from build123d import *

# Parameters (mm, degrees)
ESBO_O1_R                = 12.1
ESBO_O1_R_2              = 1.6
RESSALTO_EXTRUS_O1_DEPTH = 6
FILETE2_R                = 5
FILETE3_R                = 4


with BuildPart() as part:
    # Esboço1 → Ressalto-extrusão1 (new body)
    with BuildSketch(Plane.XY):
        with BuildLine():
            Line((-25, 4), (-16.625582697, 4))
            ThreePointArc((-16.625582697, 4), (0, 17.1), (16.625582697, 4))
            Line((16.625582697, 4), (25, 4))
            Line((25, 4), (25, -4))
            Line((25, -4), (16.625582697, -4))
            ThreePointArc((16.625582697, -4), (0, -17.1), (-16.625582697, -4))
            Line((-16.625582697, -4), (-25, -4))
            Line((-25, -4), (-25, 4))
        make_face()
        Circle(ESBO_O1_R, mode=Mode.SUBTRACT)
        with Locations((-21, 0)):
            Circle(ESBO_O1_R_2, mode=Mode.SUBTRACT)
        with Locations((21, 0)):
            Circle(ESBO_O1_R_2, mode=Mode.SUBTRACT)
    extrude(amount=RESSALTO_EXTRUS_O1_DEPTH)

    # Filete2
    filete2_edges = [part.edges().sort_by_distance(p)[0] for p in [
        (-16.625582697, 4, 3),
        (16.625582697, 4, 3),
        (16.625582697, -4, 3),
        (-16.625582697, -4, 3),
    ]]
    fillet(filete2_edges, radius=FILETE2_R)

    # Filete3
    filete3_edges = [part.edges().sort_by_distance(p)[0] for p in [
        (25, -4, 3),
        (25, 4, 3),
        (-25, -4, 3),
        (-25, 4, 3),
    ]]
    fillet(filete3_edges, radius=FILETE3_R - 0.0001)  # a hair under: the kernel refuses the full size


solid = part.part
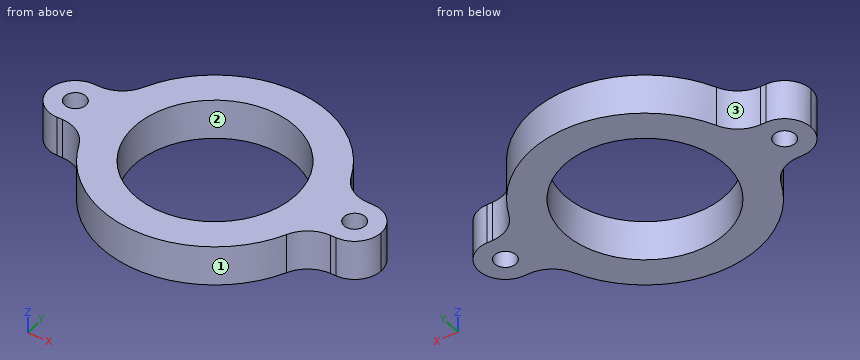
Could you check a few things on this model? Use its own coordinates, in mm. Face numbers are marked on the shaded views. Give positions to 0.01 mm unless a question says otherwise; leave off trailing zeros. Order: outer loops, then holes, each group sorted by start corner. A loop starts at its lowest first (then second) coordinate and runs counter-clockwise, first axis right, second up.
1. Thinking about a two-plate mould opening in Y: for the marked faces 1, 2 and 3, which applies, +Y half, -Y half, draft (parallel to the pull), parting line (faces both ways), or undercut?
Answers below:
face 1: -Y half
face 2: undercut
face 3: +Y half
2. For pin 1 (0.7 mm diameter, centred on x = 21, z = 2, fed in from +Y); pin 2 (1 mm diameter, centred on x = 5.5, z = 1, fed in from -Y); pin 3 (0.7 mm diameter, centred on x = -21, z = 2, fed in from -Y); pin 4 (4 mm diameter, centred on x = -21, y = 0, fed in from +Z), each with a flat end and sliding along its axis, tell me the tip position at first contact or that it passes through.
Answers below:
pin 1: stops at y = 4
pin 2: stops at y = -16.35
pin 3: stops at y = -4
pin 4: stops at z = 6
3. Suppose I cut it at B-B (x = 9). Write out the boundary of the cut face in (y, z).
Answers below:
outline: (-14.54, 0) - (-8.09, 0) - (-8.09, 6) - (-14.54, 6) - close; (8.09, 0) - (14.54, 0) - (14.54, 6) - (8.09, 6) - close
4. I need wall thicknesses on L1, parallel to Y at x = 21, z = 1.3; L2, parallel to Y at x = 0, z = 3.35; L3, parallel to X at y = -1, z = 5.1. Which ranges of each line are inside material? Lowest first, please.
Answers below:
L1: y = -4 to -1.6, 1.6 to 4
L2: y = -17.1 to -12.1, 12.1 to 17.1
L3: x = -24.87 to -22.25, -19.75 to -12.06, 12.06 to 19.75, 22.25 to 24.87
5. Suppose I cut it at A-A (z = 4.7). State how many separate pieces and enclosed holes the cut face has, plus the area to 3 significant figures.
Answers below:
separate pieces: 1
enclosed holes: 3
area: 566 mm2
6. Suppose I cut it at C-C (y = 9.5). Write out the boundary of the cut face in (x, z).
Answers below:
outline: (-14.22, 0) - (-7.49, 0) - (-7.49, 6) - (-14.22, 6) - close; (7.49, 0) - (14.22, 0) - (14.22, 6) - (7.49, 6) - close
